Geometry check sheet. Reference: the model listing, model coordinates, mm. A direction names the side the tool comes from. Give positions to 0.01 mm unless a question says otherwise; leave off trailing zeros. Order: outer loops, then holes, each group sorted by start corner. A loop starts at its lowest first (then second) coordinate and runs counter-clockwise, first axis right, second up.
Autodesk Inventor part; units mm, degrees
ref_plane "YZ Plane" through (0, 0, 0) normal (1, 0, 0) x (0, 1, 0)
ref_plane "XZ Plane" through (0, 0, 0) normal (0, 1, 0) x (-1, 0, 0)
ref_plane "XY Plane" through (0, 0, 0) normal (0, 0, 1) x (1, 0, 0)
sketch "Sketch1" plane through (0, 0, 0) normal (0, 1, 0) x (-1, 0, 0)
  circle A0 centre (0, 0) radius 11
  circle A1 centre (0, 0) radius 13.1577
  dimension "d0" = 22
  dimension "d40" = 26.3154
extrude "Extrusion1" add sketch "Sketch1" along normal blind 17 contours A0
hole "Hole1" at (0, 0, 0) direction (0, 1, 0) diameter 21 depth 7.5
ref_plane "Work Plane1" through (0, 12.25, 0) normal (0, -1, 0) x (1, 0, 0)
sketch "Sketch2" plane through (0, 7.5, 0) normal (0, -1, 0) x (1, 0, 0)
  circle A0 centre (0, 0) radius 3.5
  line L0 (0, 0) -> (2, 0) construction
  line L1 (0, 0) -> (2, 0) construction
  dimension "d10" = 7
extrude "Extrusion2" add sketch "Sketch2" along normal blind 5
sketch "Sketch3" plane through (0, 2.5, 0) normal (0, -1, 0) x (1, 0, 0)
  line L0 (0, 0) -> (-0.875, -1.5155)
  line L1 (0, 0) -> (1.75, 0) construction
  line L2 (0, 0) -> (-0.875, 1.5155)
  dimension "d19" = 1.75
  dimension "d20" = 120
  dimension "d21" = 1.75
hole "Hole2" at (-0.875, 2.5, -1.5155) at (-0.875, 2.5, 1.5155) direction (0, 1, 0) diameter 1.6 depth 24
hole "Hole3" at (1.75, 2.5, 0) direction (0, 1, 0) diameter 1.8 depth 23.25
ref_plane "Work Plane2" through (0, 12.25, 0) normal (0, 1, 0) x (1, 0, 0)
extrude "Extrusion3" add sketch "Sketch1" along normal blind 17
extrude "Extrusion4" cut sketch "Sketch1" along normal blind 8.25
sketch "Sketch4" plane through (0, 17, 0) normal (0, 1, 0) x (1, 0, 0)
  circle A0 centre (0, 0) radius 13.1577
  circle A1 centre (0, 0) radius 10
extrude "Extrusion5" cut sketch "Sketch4" against normal blind 7.5
sketch "Sketch5" plane through (0, 9.5, 0) normal (0, 1, 0) x (1, 0, 0)
  circle A0 centre (0, 0) radius 13.1577
  arc A1 (0, -13.1577) -> (13.1577, 0) centre (0, 0) ccw
  line L0 (13.1577, 0) -> (10, 0)
  circle A2 centre (0, 0) radius 10
  arc A3 (0, 13.1577) -> (-13.1577, 0) centre (0, 0) ccw
  line L1 (-13.1577, 0) -> (-10, 0)
  line L2 (0, 13.1577) -> (0, 10)
  arc A4 (0, -10) -> (10, 0) centre (0, 0) ccw
  arc A5 (0, 10) -> (-10, 0) centre (0, 0) ccw
  line L3 (0, -13.1577) -> (0, -10)
extrude "Extrusion6" cut sketch "Sketch5" against normal blind 1.25 contours A0 L3 A2 L0 | L2 A2 L1 A0
hole "Hole4" at (1.75, 2.5, 0) direction (0, 1, 0) diameter 2.2 depth 2.3
hole "Hole5" at (-0.875, 2.5, 1.5155) at (-0.875, 2.5, -1.5155) direction (0, 1, 0) diameter 1.9 depth 2.3
properties part number "cap"
Q1. Access from +Z, -Z, +X, -X, +Y, -Y to the whole of each face (thin tool, end or side, straight path). Record for faces 1 (the face through (8, 8.25, -8)), 2 (the face through (-12, 9, 0)), 3 (the face through (0, 2.5, 0)), 4 (the face through (7, 8.25, 8)).
Q2. Cross-section at C-C, the plane z = 4.5. Record the boundary of the cut face in (x, y), and give its area (3 significant figures).
Q3. Cross-section at B-B, the plane x = 1.75. Record the boundary of the cut face in (y, z), and give its area (3 significant figures).
Q4. Gauge pin test, flat ends, axial feed: P1, Ø5, axis at x = -0.5, y = 2, coming from the +Z side; P2, Ø7.5, axis at x = 1, z = -0.5, coming from the -Y side; P3, Ø0.7, axis at x = 2, z = 0, coming from the -Y side; P4, Ø6, axis at x = 5, y = 14.5, coming from the -Z side. Record the tip position at first contact, or that the pin passes through.
Q5. Release check for a two-part mould opening along X. For faces 5 (the face through (0.66, 3.67, 0.14)), 6 (the face through (0, 9, -12)), 7 (the face through (-7.2, 8.25, -7.2)) record: pulls with the +X half, pulls with the -X half, needs draft (parallel to the pull), parting line crosses it, or undercut.
Q6. Cross-section at D-D, the plane y = 2. Record the boundary of the cut face in (x, z), and give its area (3 significant figures).
Q7. Cross-section at A-A, the plane y = 4. Give the number of separate pieces and of enclosed holes in the cut face, and give its area (3 significant figures).
Q8. Thickness scan on L1, parallel to Z at x = 0, y = 6.25; L2, parallel to X at y = 8, z = 0; L3, parallel to Z at x = 1, y = 6. Record the ranges inside material, lowest first.
Answers follow:
1. face 1: -Z, +X, -Y
1. face 2: -Z, -X, +Y
1. face 3: -Y
1. face 4: +Z, +X, +Y
2. outline: (-12.36, 8.25) - (-10.04, 8.25) - (-10.04, 0) - (-9.49, 0) - (-9.49, 7.5) - (9.49, 7.5) - (9.49, 0) - (10.04, 0) - (10.04, 8.25) - (8.93, 8.25) - (8.93, 17) - (-8.93, 17) - (-8.93, 9.5) - (-12.36, 9.5) - close
2. area: 184 mm2
3. outline: (0, -10.86) - (8.25, -10.86) - (8.25, -13.04) - (9.5, -13.04) - (9.5, -9.85) - (17, -9.85) - (17, -0.9) - (4.8, -0.9) - (4.8, -1.1) - (2.5, -1.1) - (2.5, -3.03) - (7.5, -3.03) - (7.5, -10.35) - (0, -10.35) - close; (0, 10.35) - (7.5, 10.35) - (7.5, 3.03) - (2.5, 3.03) - (2.5, 1.1) - (4.8, 1.1) - (4.8, 0.9) - (17, 0.9) - (17, 9.85) - (8.25, 9.85) - (8.25, 10.86) - (0, 10.86) - close
3. area: 203 mm2
4. P1: stops at z = 11
4. P2: stops at y = 2.5
4. P3: passes through
4. P4: stops at z = -9.8
5. face 5: undercut
5. face 6: pulls with the -X half
5. face 7: needs draft
6. outline: circle Ø22 at (0, 0); hole circle Ø21 at (0, 0)
6. area: 33.8 mm2
7. separate pieces: 2
7. enclosed holes: 4
7. area: 62.8 mm2
8. L1: z = -11 to -10.5, -3.5 to 3.5, 10.5 to 11
8. L2: x = -11 to 0.85, 2.65 to 11
8. L3: z = -10.95 to -10.45, -3.35 to -0.5, 0.5 to 3.35, 10.45 to 10.95
